Could you check a few things on this model? Use its own coordinates, in mm. Face numbers are marked on the shaded views. Give positions to 0.01 mm unless a question says otherwise; leave off trailing zeros. Loops run counter-clockwise (first coordinate to the right, second up) from the corner with the lowest first, then second, coordinate; pieces in that order, holes last. Notation, with made-up numbers: (-9.5, 75) - (44.5, 75) arc R20 cw to (44.5, 97) - close; hole circle Ø6 at (86.25, 72). An arc over 180 degrees is marked (long way). Write each question's results on one line, items separated by ' | '. Start each with the question number.
1) I want a section at A-A, the plane z = 0. Write out the boundary of the cut face in (x, y).
2) If we mould it in two halves opening along Z, with no side actions, what happens to the marked faces 1, 2 and 3? For each: +Z half, -Z half, draft (parallel to the pull), parting line (faces both ways), or undercut.
3) If I drill on probe 1 along X at (y, z) = (5.75, 0); probe 2 along Y at (x, z) = (-42, 0); probe 3 along Z at (x, y) = (-17.5, 11.75), over which ranges is the centre line in solid material (lowest first)? Write a range as [from, to].
4) I want a section at D-D, the plane x = -14.5. Write out the boundary of the cut face in (y, z), and give its area (3 significant figures).
5) I'm going to push flat-ended pins straight in: pin 1 (6 mm diameter, centred on y = 8, z = 34.5, fed in from -X); pin 2 (4 mm diameter, centred on x = 23.5, y = 7.5, fed in from -Z); pin 3 (8 mm diameter, centred on y = 12, z = -29, fed in from +X); pin 4 (6 mm diameter, centred on x = 24.5, z = 26.5, fed in from -Y). Where does each tip first touch, or does it pass through?
6) I want a section at B-B, the plane x = 0. Write out the boundary of the cut face in (y, z).
7) I want a section at C-C, the plane y = 8. Write out the boundary of the cut face in (x, z) (1 decimal).
from build123d import *

# Parameters (mm, degrees)
SKETCH1_R           = 46.0375
SKETCH1_R_2         = 39.6875
BOSS_EXTRUDE1_DEPTH = 19.05
SKETCH4_R           = 3.175
CUT_EXTRUDE1_DEPTH  = 76.2
SKETCH5_R           = 3.175
CUT_EXTRUDE2_DEPTH  = 76.2
SKETCH3_R           = 3.175
CUT_EXTRUDE3_DEPTH  = 76.2


with BuildPart() as part:
    # Sketch1 → Boss-Extrude1 (new body)
    with BuildSketch(Plane(origin=(0, 0, 0), x_dir=(1, 0, 0), z_dir=(0, 1, 0))):
        with Locations(Location((0, 0, 0), (0, 0, 90))):
            Circle(SKETCH1_R)
        with Locations(Location((0, 0, 0), (0, 0, 90))):
            Circle(SKETCH1_R_2, mode=Mode.SUBTRACT)
    extrude(amount=BOSS_EXTRUDE1_DEPTH)

    # Sketch4 → Cut-Extrude1 (cut)
    with BuildSketch(Plane(origin=(0, 0, 0), x_dir=(0.8660254037844364, 0, 0.500000000000004), z_dir=(-0.500000000000004, 0, 0.8660254037844365))):
        with Locations((0, 9.525)):
            Circle(SKETCH4_R)
    extrude(amount=-CUT_EXTRUDE1_DEPTH, mode=Mode.SUBTRACT)

    # Sketch5 → Cut-Extrude2 (cut)
    with BuildSketch(Plane(origin=(0, 0, 0), x_dir=(-0.8660254037844363, 0, 0.5000000000000043), z_dir=(-0.5000000000000043, 0, -0.8660254037844363))):
        with Locations((0, 9.525)):
            Circle(SKETCH5_R)
    extrude(amount=-CUT_EXTRUDE2_DEPTH, mode=Mode.SUBTRACT)

    # Sketch3 → Cut-Extrude3 (cut)
    with BuildSketch(Plane(origin=(0, 0, 0), x_dir=(0, 0, -1), z_dir=(1, 0, 0))):
        with Locations((0, 9.525)):
            Circle(SKETCH3_R)
    extrude(amount=-CUT_EXTRUDE3_DEPTH, mode=Mode.SUBTRACT)


solid = part.part
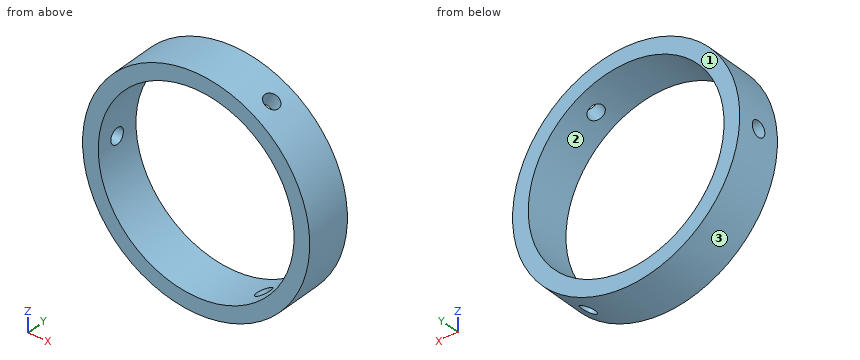
Answers:
1) outline: (-46.04, 0) - (-39.69, 0) - (-39.69, 6.35) - (-46.04, 6.35) - close; (-46.04, 12.7) - (-39.69, 12.7) - (-39.69, 19.05) - (-46.04, 19.05) - close; (39.69, 0) - (46.04, 0) - (46.04, 19.05) - (39.69, 19.05) - close
2) face 1: draft | face 2: undercut | face 3: parting line
3) probe 1: x = [-46.04, -39.69], [39.69, 46.04] | probe 2: y = [0, 6.35], [12.7, 19.05] | probe 3: z = [-42.58, -35.62], [35.62, 42.58]
4) outline: (0, -43.69) - (19.05, -43.69) - (19.05, -36.94) - (0, -36.94) - close; (0, 36.94) - (19.05, 36.94) - (19.05, 43.69) - (0, 43.69) - close | area: 257 mm2
5) pin 1: stops at x = -33.57 | pin 2: stops at z = -40.64 | pin 3: stops at x = 38.66 | pin 4: passes through
6) outline: (0, -46.04) - (19.05, -46.04) - (19.05, -39.69) - (0, -39.69) - close; (0, 39.69) - (19.05, 39.69) - (19.05, 46.04) - (0, 46.04) - close
7) outline: (-46, -2.8) arc R46 ccw to (20.6, -41.2) - (17.4, -35.7) arc R39.7 cw to (-39.6, -2.8) - close; (-46, 2.8) - (-39.6, 2.8) arc R39.7 cw to (17.4, 35.7) - (20.6, 41.2) arc R46 ccw to start; (22.2, -32.9) - (25.4, -38.4) arc R46 ccw to (25.4, 38.4) - (22.2, 32.9) arc R39.7 cw to start
